from build123d import *

# Parameters (mm, degrees)
ESQUISSE1_W             = 50
ESQUISSE1_H             = 50
ESQUISSE1_R             = 1.7
BOSS_EXTRU_1_DEPTH      = 3
ESQUISSE2_W             = 50
ESQUISSE2_H             = 20
ESQUISSE2_R             = 2.5
BOSS_EXTRU_2_DEPTH      = 3
BOSS_EXTRU_3_DEPTH      = 1.5
BOSS_EXTRU_3_DEPTH_BACK = 1.5
ESQUISSE5_W             = 8
ESQUISSE5_H             = 17
ENL_V_MAT_EXTRU_2_DEPTH = 10
CONG_1_R                = 3
CONG_2_R                = 3
CONG_3_R                = 2
ESQUISSE4_W             = 20
ESQUISSE4_H             = 30
ENL_V_MAT_EXTRU_1_DEPTH = 73.725511411
CONG_4_R                = 3


with BuildPart() as part:
    # Esquisse1 → Boss.-Extru.1 (new body)
    with BuildSketch(Plane(origin=(0, 0, 0), x_dir=(1, 0, 0), z_dir=(0, 1, 0))):
        with Locations((25, 25)):
            Rectangle(ESQUISSE1_W, ESQUISSE1_H)
        with Locations(Location((5, 5, 0), (0, 0, 270))):
            Circle(ESQUISSE1_R, mode=Mode.SUBTRACT)
        with Locations(Location((5, 45, 0), (0, 0, 90))):
            Circle(ESQUISSE1_R, mode=Mode.SUBTRACT)
        with Locations(Location((45, 45, 0), (0, 0, 270))):
            Circle(ESQUISSE1_R, mode=Mode.SUBTRACT)
        with Locations(Location((45, 5, 0), (0, 0, 90))):
            Circle(ESQUISSE1_R, mode=Mode.SUBTRACT)
    extrude(amount=BOSS_EXTRU_1_DEPTH)

    # Esquisse2 → Boss.-Extru.2 (add)
    with BuildSketch(Plane.XY):
        with Locations((25, 10)):
            Rectangle(ESQUISSE2_W, ESQUISSE2_H)
        with Locations((15, 10)):
            Circle(ESQUISSE2_R, mode=Mode.SUBTRACT)
        with Locations(Location((35, 10, 0), (0, 0, 180))):
            Circle(ESQUISSE2_R, mode=Mode.SUBTRACT)
    extrude(amount=BOSS_EXTRU_2_DEPTH)

    # Esquisse3 → Boss.-Extru.3 (add, two sides: drawn at the far end of the back side and taken through both)
    with BuildSketch(Plane(origin=(25, 0, 0), x_dir=(0, 0, -1), z_dir=(1, 0, 0)).offset(-BOSS_EXTRU_3_DEPTH_BACK)):
        Polygon((0, 20), (3, 20), (50, 6), (50, 3), (0, 3), align=None)
    extrude(amount=BOSS_EXTRU_3_DEPTH + BOSS_EXTRU_3_DEPTH_BACK)

    # Esquisse5 → Enlèv. mat.-Extru.2 (cut)
    with BuildSketch(Plane(origin=(0, 0, 0), x_dir=(-1, 0, 0), z_dir=(0, 0, -1))):
        with Locations((-4, 11.5)):
            Rectangle(ESQUISSE5_W, ESQUISSE5_H)
        with Locations((-46, 11.5)):
            Rectangle(ESQUISSE5_W, ESQUISSE5_H)
    extrude(amount=-ENL_V_MAT_EXTRU_2_DEPTH, mode=Mode.SUBTRACT)

    # Congé1
    cong_1_edges = [part.edges().sort_by_distance(p)[0] for p in [
        (0, 1.5, -50),
        (50, 1.5, -50),
    ]]
    fillet(cong_1_edges, radius=CONG_1_R)

    # Congé2
    cong_2_edges = [part.edges().sort_by_distance(p)[0] for p in [
        (25, 20, -3),
        (25, 6, -50),
        (42, 20, 1.5),
        (8, 20, 1.5),
        (8, 3, 1.5),
        (42, 3, 1.5),
    ]]
    fillet(cong_2_edges, radius=CONG_2_R)

    # Congé3
    cong_3_edges = [part.edges().sort_by_distance(p)[0] for p in [
        (26.5, 11.5, 0),
    ]]
    fillet(cong_3_edges, radius=CONG_3_R)
    cong_3_2_edges = [part.edges().sort_by_distance(p)[0] for p in [
        (36.75, 3, 0),
    ]]
    fillet(cong_3_2_edges, radius=CONG_3_R)
    cong_3_3_edges = [part.edges().sort_by_distance(p)[0] for p in [
        (23.5, 11.5, 0),
    ]]
    fillet(cong_3_3_edges, radius=CONG_3_R)
    cong_3_4_edges = [part.edges().sort_by_distance(p)[0] for p in [
        (23.5, 3, -26),
    ]]
    fillet(cong_3_4_edges, radius=CONG_3_R)

    # Esquisse4 → Enlèv. mat.-Extru.1 (cut, through all)
    with BuildSketch(Plane(origin=(0, 3, 0), x_dir=(1, 0, 0), z_dir=(0, 1, 0))):
        with Locations((40, 25)):
            Rectangle(ESQUISSE4_W, ESQUISSE4_H)
        with Locations((10, 25)):
            Rectangle(ESQUISSE4_W, ESQUISSE4_H)
    extrude(amount=-ENL_V_MAT_EXTRU_1_DEPTH, mode=Mode.SUBTRACT)

    # Congé4
    cong_4_edges = [part.edges().sort_by_distance(p)[0] for p in [
        (50, 1.5, -40),
        (50, 1.5, -10),
        (30, 1.5, -10),
        (30, 1.5, -40),
        (20, 1.5, -10),
        (0, 1.5, -10),
        (0, 1.5, -40),
        (20, 1.5, -40),
    ]]
    fillet(cong_4_edges, radius=CONG_4_R)


solid = part.part
Model file for the job. Use its own axes, mm. A direction names the side the tool comes from. Give positions to 0.01 mm unless a question says otherwise; leave off trailing zeros. Order: outer loops, then holes, each group sorted by start corner. A loop starts at its lowest first (then second) coordinate and runs counter-clockwise, first axis right, second up. Notation, with made-up numbers: (38.5, 86.25) -> (68.5, 86.25) arc R20 cw to (68.5, 117.25) -> close; hole circle Ø6 at (-22.5, 52). An arc over 180 degrees is marked (long way). Use CSV: the item, a comma, the result in double quotes.
1. Band-saw the part on A-A, the plane x = 15. Give the cut face in (y, z), then the cut area to 3 significant figures.
Outcome:
outline,"(0, -50) -> (3, -50) -> (3, -40) -> (0, -40) -> close; (0, -10) -> (3, -10) -> (3, -2) arc R2 cw to (5, 0) -> (7.5, 0) -> (7.5, 3) -> (0, 3) -> close; (12.5, 0) -> (20, 0) -> (20, 3) -> (12.5, 3) -> close"
area,"106 mm²"
2. 3-axis set-ups, long thin cutter, end or side, ignore diameter. For faces 1 (the cylindrical face through (13.13, 3.57, -0.6)), 2 (the flat face through (40, 2, -10)), 3 (the flat face through (8, 11, 1)): which of +Z, -Z, +X, -X, +Y, -Y reach the whole face in a straight line?
Outcome:
face 1,"-Z, -X, +Y"
face 2,"+X, +Y, -Y"
face 3,"+Z, -Z, -X, +Y"
3. Band-saw the part on D-D, the plane z = -24.5. Give the cut face in (x, y), then the cut area to 3 significant figures.
Outcome:
outline,"(20, 0) -> (30, 0) -> (30, 3) -> (28.5, 3) arc R2 cw to (26.5, 5) -> (26.5, 13.6) -> (23.5, 13.6) -> (23.5, 5) arc R2 cw to (21.5, 3) -> (20, 3) -> close"
area,"63.5 mm²"
4. Mould opens along Z. For faces 4 (the flat face through (42, 11, 1)), 5 (the cylindrical face through (4.93, 1.48, -43.3)), 6 (the cylindrical face through (49.14, 1.48, -9.1)), 7 (the cylindrical face through (27.1, 12.6, -0.57)) say: +Z half, -Z half, draft (parallel to the pull), parting line (faces both ways), or undercut.
Outcome:
face 4,"draft"
face 5,"undercut"
face 6,"undercut"
face 7,"-Z half"
5. Band-saw the part on C-C, the plane y = 9.25. Give the cut face in (x, z).
Outcome:
outline,"(8, 0) -> (12.62, 0) -> (12.62, 3) -> (8, 3) -> close; (17.38, 0) -> (21.5, 0) arc R2 cw to (23.5, -2) -> (23.5, -39.09) -> (26.5, -39.09) -> (26.5, -2) arc R2 cw to (28.5, 0) -> (32.62, 0) -> (32.62, 3) -> (17.38, 3) -> close; (37.38, 0) -> (42, 0) -> (42, 3) -> (37.38, 3) -> close"
6. Drill centre lines: line 1 along X through (y, z) = (1.2, -5); line 2 along X through (y, z) = (11.75, 0.5); line 3 along Y through (x, z) = (31, -47). Where is each one in solid material? Low to high. Write a range as from..to.
Outcome:
line 1,"0..3.3, 6.7..43.3, 46.7..50"
line 2,"8..13.21, 16.79..33.21, 36.79..42"
line 3,"0..3"
7. Drop flat-ended pins along their axis: pin 1 (23.5 mm diameter, centred on x = 42, z = -17, fed in from +Y); pin 2 (2 mm diameter, centred on y = 5, z = -40.5, fed in from -X); pin 3 (1.5 mm diameter, centred on y = 2, z = -23.5, fed in from -X); pin 4 (3 mm diameter, centred on x = 5, z = -45, fed in from +Y). Give the stop position or say it passes through.
Outcome:
pin 1,"y = 3"
pin 2,"x = 23.23"
pin 3,"x = 20"
pin 4,"through"
8. Band-saw the part on B-B, the plane z = -6. Give the cut face in (x, y).
Outcome:
outline,"(0, 0) -> (3.63, 0) -> (3.63, 3) -> (0, 3) -> close; (6.37, 0) -> (43.63, 0) -> (43.63, 3) -> (28.5, 3) arc R2 cw to (26.5, 5) -> (26.5, 19.11) -> (23.5, 19.11) -> (23.5, 5) arc R2 cw to (21.5, 3) -> (6.37, 3) -> close; (46.37, 0) -> (50, 0) -> (50, 3) -> (46.37, 3) -> close"
